Check sheet for the modelled part. Datum: model origin and axes. Units: mm. A direction names the side the tool comes from. Round coordinates to 2 decimals unless told otherwise and drop trailing zeros. Order: outer loops, then holes, each group sorted by start corner. A loop starts at its lowest first (then second) coordinate and runs counter-clockwise, first axis right, second up.
(1) Sectioned sample at B-B, the plane y = 0. Enter the section's corners in (x, z), and give its area (3 significant figures).
(2) Mould release check, pull along X, two halves, no side actions. Record for faces 6 (the flat face through (-2.1, 0, 8)), 7 (the flat face through (-7.5, 0, 11)), 8 (the flat face through (-13, 19, 0)), 9 (the flat face through (-20, 11, 5.5)): released by +X, released by -X, zero draft, split by the parting line, or undercut.
(3) Thickness scan on probe 1 along Y at (x, z) = (0, 1.95); probe 2 along Y at (x, z) = (0, 6.4); probe 3 along X at (y, z) = (11, 3.25). Record the ranges inside material, lowest first.
(4) Sectioned sample at D-D, the plane y = 25. Enter the section's corners in (x, z).
(5) Sectioned sample at A-A, the plane z = 10.5. Enter the section's corners in (x, y), and give its area (3 significant figures).
(6) Sectioned sample at C-C, the plane z = 2. Enter the section's corners in (x, y).
(7) Depth check by flat-ended pin: pin 1 (2.5 mm diameter, centred on y = 7, z = 11.5, fed in from -X); pin 2 (1 mm diameter, centred on x = -16, y = 13, fed in from -Z); pin 3 (2 mm diameter, centred on y = 5, z = 4.5, fed in from -X); pin 4 (2.5 mm diameter, centred on x = 21.65, y = 12.5, fed in from -Z). Enter the tip coordinate at first touch or a pass-through.
(8) Tool access check on faces 1 (the cylindrical face through (26.327, 10.916, 3.451)), 2 (the cylindrical face through (-0.65, 22.07, 6.26)), 3 (the flat face through (3, 0, 12.2)), 4 (the flat face through (7.5, 0, 11)), 5 (the flat face through (5, 18, 11)). Record the directions out of +Z, -Z, +X, -X, +Y, -Y that give a thin tool (end or side, any length) a straight path to the whole face; none if there is none.
Autodesk Inventor part; units mm, degrees
ref_plane "YZ Plane" through (0, 0, 0) normal (1, 0, 0) x (0, 1, 0)
ref_plane "XZ Plane" through (0, 0, 0) normal (0, 1, 0) x (-1, 0, 0)
ref_plane "XY Plane" through (0, 0, 0) normal (0, 0, 1) x (1, 0, 0)
sketch "スケッチ1" plane through (0, 0, 0) normal (0, 0, 1) x (1, 0, 0)
  circle A0 centre (0, 0) radius 28.5
  circle A1 centre (0, 0) radius 20
  dimension "d0" = 57
  dimension "d1" = 40
extrude "押し出し1" add sketch "スケッチ1" along normal blind 10 contours A0 | A1
sketch "スケッチ2" plane through (0, 0, 0) normal (0, 0, -1) x (-1, 0, 0)
  circle A0 centre (0, 0) radius 22.5
  dimension "d4" = 45
extrude "押し出し2" cut sketch "スケッチ2" against normal blind 5
sketch "スケッチ4" plane through (0, 0, 10) normal (0, 0, 1) x (1, 0, 0)
  circle A0 centre (0, 0) radius 25
  circle A1 centre (0, -25) radius 1.7
  circle A2 centre (21.6506, -12.5) radius 1.7
  circle A3 centre (21.6506, 12.5) radius 1.7
  circle A4 centre (0, 25) radius 1.7
  circle A5 centre (-21.6506, 12.5) radius 1.7
  circle A6 centre (-21.6506, -12.5) radius 1.7
  dimension "d15" = 50
  dimension "d16" = 3.4
  dimension "d19" = 360
extrude "押し出し4" cut sketch "スケッチ4" against normal blind 10 contours A3 A0 | A0 A3 | A2 A0 | A0 A2 | A4 A0 | A0 A4 | A1 A0 | A0 A1 | A5 A0 | A0 A5 | A6 A0 | A0 A6
sketch "スケッチ5" plane through (0, 0, 10) normal (0, 0, 1) x (1, 0, 0)
  circle A0 centre (0, 0) radius 28.5
extrude "押し出し5" cut sketch "スケッチ5" against normal blind 3
sketch "スケッチ6" plane through (0, 0, 7) normal (0, 0, 1) x (1, 0, 0)
  circle A0 centre (0, 0) radius 21.5
  circle A1 centre (0, 25) radius 1.7
  circle A2 centre (0, 25) radius 3
  circle A3 centre (-21.6506, 12.5) radius 3
  circle A4 centre (-21.6506, -12.5) radius 3
  circle A5 centre (0, -25) radius 3
  circle A6 centre (21.6506, -12.5) radius 3
  circle A7 centre (21.6506, 12.5) radius 3
  dimension "d25" = 43
  dimension "d26" = 6
  dimension "d29" = 360
extrude "押し出し6" cut sketch "スケッチ6" against normal blind 1.5 contours A1 | A2 | A3 | A4 | A5 | A6 | A7
sketch "スケッチ7" plane through (0, 0, 7) normal (0, 0, 1) x (1, 0, 0)
  line L0 (0, 0) -> (7.5, 0)
  line L1 (7.5, 0) -> (7.5, 18)
  line L2 (7.5, 18) -> (-7.5, 18)
  line L3 (-7.5, 18) -> (-7.5, -18)
  line L4 (-7.5, -18) -> (7.5, -18)
  line L5 (7.5, -18) -> (7.5, 0)
  dimension "d33" = 7.5
  dimension "d34" = 18
  dimension "d35" = 15
  dimension "d36" = 36
extrude "押し出し7" add sketch "スケッチ7" along normal blind 7
sketch "スケッチ8" plane through (-7.5, 18, 7) normal (0, 1, 0) x (1, 0, 0)
  line L0 (15, 0) -> (0, 0)
  line L1 (7.5, 0) -> (9.6, 0)
  line L2 (9.6, 0) -> (9.6, -1.5)
  line L3 (9.6, -1.5) -> (5.4, -1.5)
  line L4 (5.4, -1.5) -> (5.4, 0)
  line L5 (7.5, 0) -> (5.4, 0)
  line L6 (7.5, -1.5) -> (11.65, -1.5)
  line L7 (11.65, -1.5) -> (11.65, -5.2)
  line L8 (11.65, -5.2) -> (3.35, -5.2)
  line L9 (3.35, -5.2) -> (3.35, -1.5)
  line L10 (3.35, -1.5) -> (7.5, -1.5)
  line L11 (7.5, -5.2) -> (9.6, -5.2)
  line L12 (9.6, -5.2) -> (9.6, -7)
  line L13 (0, -7) -> (15, -7)
  line L14 (9.6, -7) -> (5.4, -7)
  line L15 (5.4, -7) -> (5.4, -5.2)
  point P0 (7.5, 7)
  dimension "d39" = 2.1
  dimension "d40" = 1.5
  dimension "d41" = 4.2
  dimension "d42" = 4.15
  dimension "d43" = 3.7
  dimension "d44" = 8.3
  dimension "d45" = 2.1
extrude "押し出し8" cut sketch "スケッチ8" against normal blind 40
fillet "フィレット1" radius 2 6 edges at (-4.8, -18, 7) (4.8, -18, 7) (7.5, 0, 7) (-7.5, 0, 7) (-4.8, 18, 7) (4.8, 18, 7)
properties part number "piper-GIM3505-8" material "ABS プラスチック"
Derived:
1. outline: (-28.5, 0) - (-22.5, 0) - (-22.5, 5) - (22.5, 5) - (22.5, 0) - (28.5, 0) - (28.5, 7) - (9.5, 7) arc R2 cw to (7.5, 9) - (7.5, 14) - (2.1, 14) - (2.1, 12.2) - (4.15, 12.2) - (4.15, 8.5) - (2.1, 8.5) - (2.1, 7) - (-2.1, 7) - (-2.1, 8.5) - (-4.15, 8.5) - (-4.15, 12.2) - (-2.1, 12.2) - (-2.1, 14) - (-7.5, 14) - (-7.5, 9) arc R2 cw to (-9.5, 7) - (-28.5, 7) - close
1. area: 236 mm2
2. face 6: undercut
2. face 7: released by -X
2. face 8: zero draft
2. face 9: undercut
3. probe 1: y = -28.5 to -26.7, -23.3 to -22.5, 22.5 to 23.3, 26.7 to 28.5
3. probe 2: y = -28.5 to -28, -22 to 22, 28 to 28.5
3. probe 3: x = -26.29 to -22.45, -20.85 to -19.63, 19.63 to 20.85, 22.45 to 26.29
4. outline: (-13.68, 0) - (-1.7, 0) - (-1.7, 5.5) - (-3, 5.5) - (-3, 7) - (-13.68, 7) - close; (1.7, 0) - (13.68, 0) - (13.68, 7) - (3, 7) - (3, 5.5) - (1.7, 5.5) - close
5. outline: (-7.5, -18) - (-4.15, -18) - (-4.15, 18) - (-7.5, 18) - close; (4.15, -18) - (7.5, -18) - (7.5, 18) - (4.15, 18) - close
5. area: 241 mm2
6. outline: circle Ø57 at (0, 0); hole circle Ø3.4 at (-21.65, -12.5); hole circle Ø3.4 at (-21.65, 12.5); hole circle Ø45 at (0, 0); hole circle Ø3.4 at (0, -25); hole circle Ø3.4 at (0, 25); hole circle Ø3.4 at (21.65, -12.5); hole circle Ø3.4 at (21.65, 12.5)
7. pin 1: stops at x = -7.5
7. pin 2: stops at z = 5
7. pin 3: stops at x = -28.22
7. pin 4: passes through
8. face 1: +Z, -Z
8. face 2: +Z
8. face 3: +Y, -Y
8. face 4: +Z, +X, +Y, -Y
8. face 5: +Z, +X, -X, +Y
